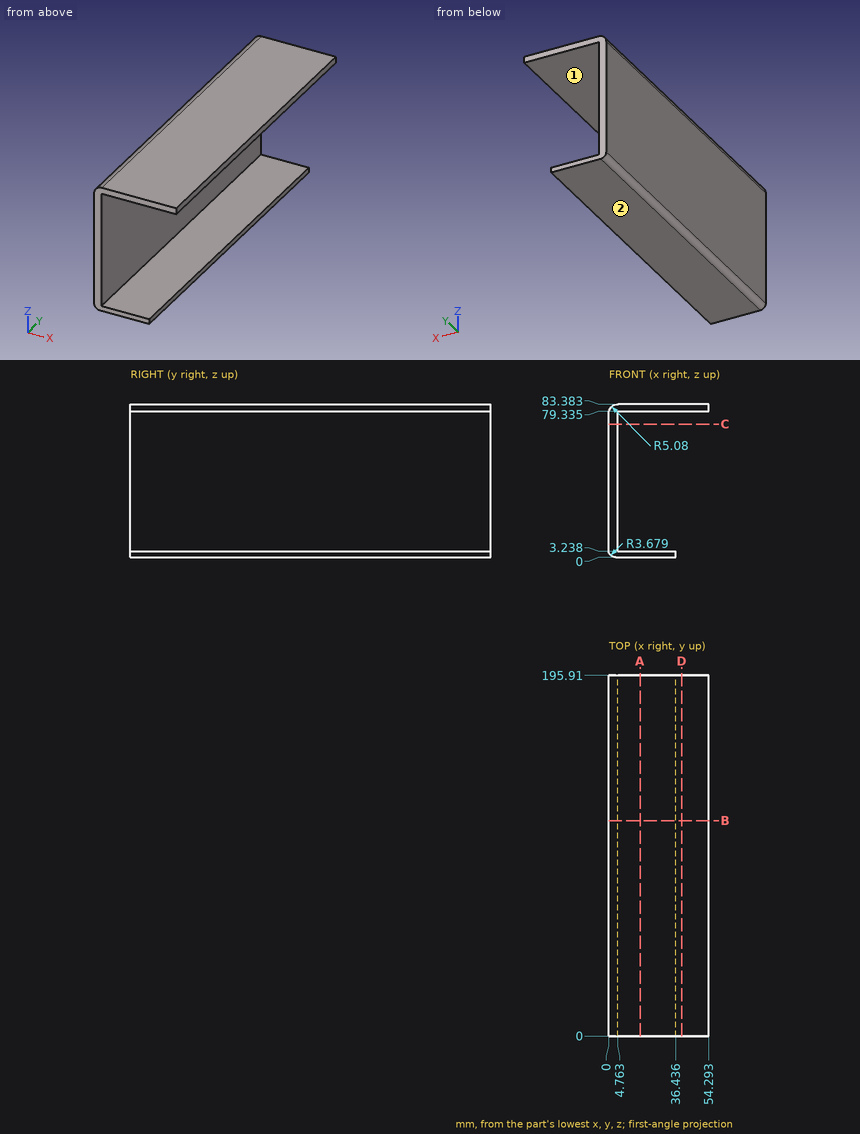
Can you work these out from the drawing? Everything is in mm from the part's minimum corner. A direction names the side the tool comes from. Give positions to 0.01 mm unless a question says otherwise; leave off trailing zeros. Order: outer loops, then holes, each group sorted by start corner. A loop starts at its lowest first (then second) coordinate and runs counter-clockwise, first axis right, second up.
1. Suppose I cut it at D-D (x = 39.5). List the corners of the cut face in (y, z) for me (1 decimal), plus the area to 3 significant figures.
2. Suppose I cut it at C-C (z = 72.5). List the corners of the cut face in (x, y) for me.
3. I need wall thicknesses on L1, parallel to Z at x = 13, y = 155 (1 decimal); L2, parallel to X at y = 54, z = 65; L3, parallel to Z at x = 4.5, y = 78. Which ranges of each line are inside material? Lowest first, please.
4. For the marked faces 1 and 2, which set-ups out of +Z, -Z, +X, -X, +Y, -Y let a thin tool reach every point of the face, with its end or its side?
5. Suppose I cut it at A-A (x = 17). List the corners of the cut face in (y, z) for me (1 decimal).
6. Will these pins go through, and if not, where does the flat tip stop? P1, Ø10, axis at y = 29.5, z = 42.5, coming from the -X side; P2, Ø1.5, axis at y = 156, z = 52, coming from the +X side; P3, Ø1.6, axis at y = 94, z = 2, coming from the +X side.
7. Suppose I cut it at B-B (y = 117). List the corners of the cut face in (x, z) for me (1 decimal).
Solved:
1. outline: (0, 79.3) - (195.9, 79.3) - (195.9, 83.4) - (0, 83.4) - close
1. area: 793 mm2
2. outline: (0, 0) - (4.76, 0) - (4.76, 195.91) - (0, 195.91) - close
3. L1: z = 0 to 3.2, 79.3 to 83.4
3. L2: x = 0 to 4.76
3. L3: z = 0 to 83.35
4. face 1: +X, +Y, -Y
4. face 2: -Z, +X, -X, +Y, -Y
5. outline: (0, 0) - (195.9, 0) - (195.9, 3.2) - (0, 3.2) - close; (0, 79.3) - (195.9, 79.3) - (195.9, 83.4) - (0, 83.4) - close
6. P1: stops at x = 0
6. P2: stops at x = 4.76
6. P3: stops at x = 36.44
7. outline: (0, 3.7) arc R3.7 ccw to (3.7, 0) - (36.4, 0) - (36.4, 3.2) - (4.8, 3.2) - (4.8, 79.3) - (54.3, 79.3) - (54.3, 83.4) - (5.1, 83.4) arc R5.1 ccw to (0, 78.3) - close
